For this review, use the dimensioned drawing (mm, ordinates from the lowest corner) and the shaded views. Round coordinates to 2 decimals unless told otherwise and drop trailing zeros. Order: outer loops, then holes, each group sorted by start corner. A loop starts at its lowest first (then second) coordinate and runs counter-clockwise, first axis right, second up. Notation, with made-up numbers: (69, 5) - (90, 5) arc R21 ccw to (90, 26) - close; hole circle Ø1 at (-22, -22.5). An arc over 180 degrees is marked (long way). Write each question's results on one line, items separated by ' | '. Start each with the question number.
(1) Take a section at C-C, the plane z = 5. Give the boundary of the cut face in (x, y).
(2) Take a section at B-B, the plane x = 5. Give the boundary of the cut face in (y, z).
(3) Insertion check: pin 1 Ø0.8 at (y, z) = (4.5, 29.5) entering from -X; pin 2 Ø0.8 at (x, y) = (29.5, 4.5) entering from +Z; pin 3 Ø1.8 at (x, z) = (54, 54) entering from +Y; pin 4 Ø3 at (x, z) = (22, 38) entering from +Y. Each pin has a flat end and moves straight along its axis. Give the tip position at first contact, or say it passes through.
(4) Take a section at A-A, the plane z = 29.5. Give the boundary of the cut face in (x, y), plus the area to 3 significant figures.
(5) For L1, parallel to X at y = 0.55, z = 6 (1 decimal); L2, parallel to X at y = 4.25, z = 50; L3, parallel to Z at x = 7, y = 4.6 (1 decimal), list the stretches that pass through material, from the lowest coordinate up. Write a range as from..to.
(6) Take a section at D-D, the plane x = 37. Give the boundary of the cut face in (y, z).
(7) Draft analysis for pull direction X (two halves, no side actions). For the marked faces 1 and 2, state which applies: pulls with the +X half, pulls with the -X half, needs draft (parallel to the pull), parting line crosses it, or undercut.
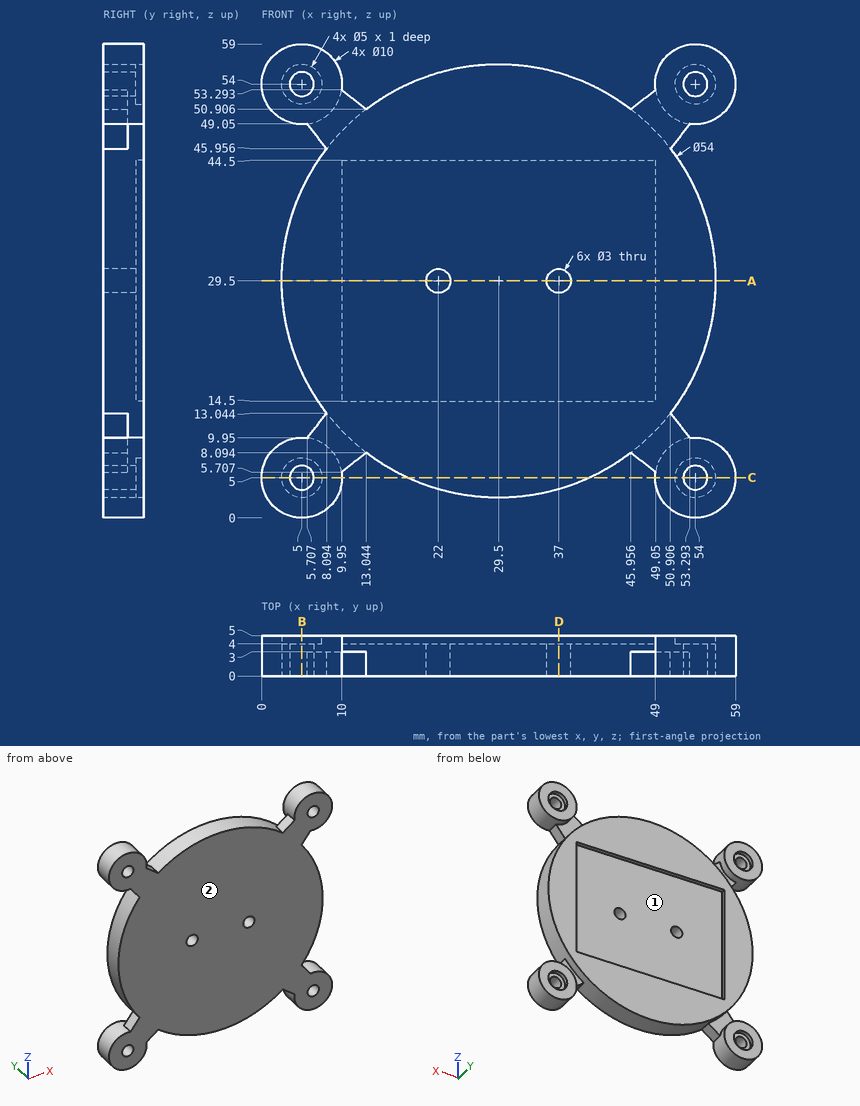
Results below:
1) outline: (0, 0) - (3.5, 0) - (3.5, 4) - (2.5, 4) - (2.5, 5) - (0, 5) - close; (6.5, 0) - (10, 0) - (10, 5) - (7.5, 5) - (7.5, 4) - (6.5, 4) - close; (18.15, 0) - (40.85, 0) - (40.85, 5) - (18.15, 5) - close; (49, 0) - (52.5, 0) - (52.5, 4) - (51.5, 4) - (51.5, 5) - (49, 5) - close; (55.5, 0) - (59, 0) - (59, 5) - (56.5, 5) - (56.5, 4) - (55.5, 4) - close
2) outline: (0, 0) - (5, 0) - (5, 2.5) - (4, 2.5) - (4, 3.5) - (0, 3.5) - close; (0, 6.5) - (4, 6.5) - (4, 7.5) - (5, 7.5) - (5, 10) - (0, 10) - close; (0, 18.15) - (5, 18.15) - (5, 40.85) - (0, 40.85) - close; (0, 49) - (5, 49) - (5, 51.5) - (4, 51.5) - (4, 52.5) - (0, 52.5) - close; (0, 55.5) - (4, 55.5) - (4, 56.5) - (5, 56.5) - (5, 59) - (0, 59) - close
3) pin 1: stops at x = 2.5 | pin 2: stops at z = 56.5 | pin 3: passes through | pin 4: stops at y = 4
4) outline: (2.5, 0) - (20.5, 0) - (20.5, 4) - (10, 4) - (10, 5) - (2.5, 5) - close; (23.5, 0) - (35.5, 0) - (35.5, 4) - (23.5, 4) - close; (38.5, 0) - (56.5, 0) - (56.5, 5) - (49, 5) - (49, 4) - (38.5, 4) - close | area: 207 mm^2
5) L1: x = 0.1..3.9, 6.1..10.3, 16.2..42.8, 48.7..52.9, 55.1..58.9 | L2: x = 2..8, 11.93..47.07, 51..57 | L3: z = 0.4..3.5, 6.5..9.6, 14.6..44.4, 49.4..52.5, 55.5..58.6
6) outline: (0, 3.56) - (5, 3.56) - (5, 14.5) - (4, 14.5) - (4, 28) - (0, 28) - close; (0, 31) - (4, 31) - (4, 44.5) - (5, 44.5) - (5, 55.44) - (0, 55.44) - close
7) face 1: undercut | face 2: needs draft
